```python
from build123d import *

# Parameters (mm, degrees)
F0_W      = 565.15
F0_H      = 1066.8
F1_DEPTH  = 19.05
F3_DEPTH  = 742.95
F5_W      = 304.8
F5_H      = 38.1
F6_DEPTH  = 88.9
F7_W      = 38.1
F7_H      = 806.45
F8_DEPTH  = 88.9
F9_W      = 346.075
F9_H      = 38.1
F10_DEPTH = 88.9
F12_W     = 304.8
F12_H     = 38.1
F13_DEPTH = 88.9
F14_W     = 177.8
F14_H     = 965.2
F15_DEPTH = 38.1


with BuildPart() as f1:
    # F0 (on Top) → F1 (new body)
    with BuildSketch(Plane.XY):
        with Locations((282.575, 533.4)):
            Rectangle(F0_W, F0_H)
    extrude(amount=F1_DEPTH)

    # F2 (on face) → F3 (join)
    with BuildSketch(Plane(origin=(0, 0, 0), x_dir=(1, 0, 0), z_dir=(0, 0, -1))):
        Polygon((130.175, -1016), (130.175, -976.3125), (130.175, -936.625), (50.8, -936.625), (50.8, -1016), align=None)
        Polygon((514.35, -1016), (514.35, -936.625), (434.975, -936.625), (434.975, -976.3125), (434.975, -1016), align=None)
        Polygon((434.975, -50.8), (434.975, -71.4375), (434.975, -109.5375), (434.975, -130.175), (514.35, -130.175), (514.35, -50.8), align=None)
        Polygon((130.175, -71.4375), (130.175, -50.8), (50.8, -50.8), (50.8, -130.175), (130.175, -130.175), (130.175, -109.5375), align=None)
    extrude(amount=F3_DEPTH)

    # F5 (on face) → F6 (join)
    with BuildSketch(Plane(origin=(0, 0, 0), x_dir=(1, 0, 0), z_dir=(0, 0, -1))):
        with Locations((282.575, -90.4875)):
            Rectangle(F5_W, F5_H)
        with Locations((282.575, -976.3125)):
            Rectangle(F5_W, F5_H)
    extrude(amount=F6_DEPTH)

    # F7 (on face) → F8 (join)
    with BuildSketch(Plane(origin=(0, 0, 0), x_dir=(1, 0, 0), z_dir=(0, 0, -1))):
        with Locations((474.6625, -533.4)):
            Rectangle(F7_W, F7_H)
        with Locations((90.4875, -533.4)):
            Rectangle(F7_W, F7_H)
    extrude(amount=F8_DEPTH)

    # F9 (on face) → F10 (join)
    with BuildSketch(Plane(origin=(0, 0, 0), x_dir=(1, 0, 0), z_dir=(0, 0, -1))):
        with Locations((282.575, -533.4)):
            Rectangle(F9_W, F9_H)
    extrude(amount=F10_DEPTH)

    # F12 (on offset) → F13 (join)
    with BuildSketch(Plane(origin=(0, 0, -590.55), x_dir=(1, 0, 0), z_dir=(0, 0, -1))):
        with Locations((282.575, -90.4875)):
            Rectangle(F12_W, F12_H)
        with Locations((282.575, -976.3125)):
            Rectangle(F12_W, F12_H)
    extrude(amount=F13_DEPTH)

    # F14 (on offset) → F15 (join)
    with BuildSketch(Plane(origin=(0, 0, -590.55), x_dir=(1, 0, 0), z_dir=(0, 0, -1))):
        with Locations((219.075, -533.4)):
            Rectangle(F14_W, F14_H)
    extrude(amount=-F15_DEPTH)


solid = f1.part
```
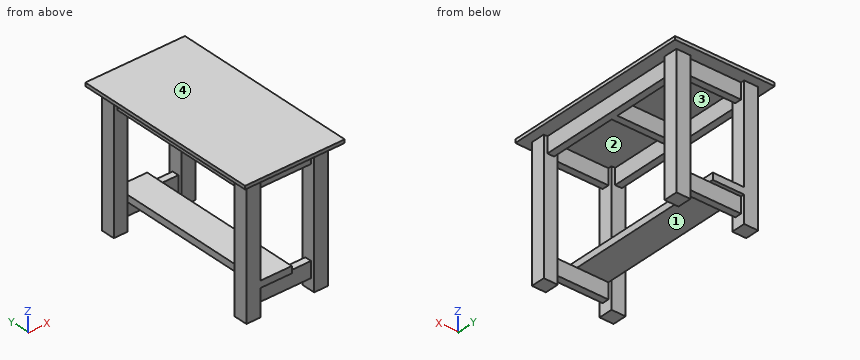
Verification items for the finished model (mm, model axes). Face numbers are marked on the shaded views. Round coordinates to 2 decimals unless told otherwise and drop trailing zeros. Write each loop counter-clockwise with the first axis right and the second up, starting at its lowest first coordinate (ties: lowest second). Pieces come first, ordered by that corner, then holes.
1. Section check B-B on z = -569. Enter the section's corners in (x, y) (3 decimals), plus the area to 3 significant figures.
2. Section check D-D on z = -291. Enter the section's corners in (x, y) (3 decimals).
3. Draft check along Z on the marked faces 1, 2, 3 and 4. Enter one of: +Z half, -Z half, draft (parallel to the pull), parting line (faces both ways), or undercut.
4. Section check A-A on x = 260.5. Enter the section's corners in (y, z).
5. Gauge pin test, flat ends, axial feed: P1, Ø10.5, axis at x = 233.5, y = 56, coming from the -Z side; P2, Ø6, axis at x = 86, z = -306, coming from the -Y side; P3, Ø24, axis at y = 89, z = -375.5, coming from the -X side. Record the tip position at first contact, or that the pin passes through.
6. Scan lines: L1, parallel to X at y = 496.5, z = -80.5; L2, parallel to Y at x = 51, z = -273 (3 decimals); L3, parallel to Z at x = 275, y = 668. Record each from-to range of solid material in increasing order.
Answer:
1. outline: (50.8, 50.8) - (307.975, 50.8) - (307.975, 1016) - (50.8, 1016) - (50.8, 936.625) - (130.175, 936.625) - (130.175, 130.175) - (50.8, 130.175) - close; (434.975, 50.8) - (514.35, 50.8) - (514.35, 130.175) - (434.975, 130.175) - close; (434.975, 936.625) - (514.35, 936.625) - (514.35, 1016) - (434.975, 1016) - close
1. area: 197,000 mm2
2. outline: (50.8, 50.8) - (130.175, 50.8) - (130.175, 130.175) - (50.8, 130.175) - close; (50.8, 936.625) - (130.175, 936.625) - (130.175, 1016) - (50.8, 1016) - close; (434.975, 50.8) - (514.35, 50.8) - (514.35, 130.175) - (434.975, 130.175) - close; (434.975, 936.625) - (514.35, 936.625) - (514.35, 1016) - (434.975, 1016) - close
3. face 1: -Z half
3. face 2: undercut
3. face 3: undercut
3. face 4: +Z half
4. outline: (0, 0) - (71.44, 0) - (71.44, -88.9) - (109.54, -88.9) - (109.54, 0) - (514.35, 0) - (514.35, -88.9) - (552.45, -88.9) - (552.45, 0) - (957.26, 0) - (957.26, -88.9) - (995.36, -88.9) - (995.36, 0) - (1066.8, 0) - (1066.8, 19.05) - (0, 19.05) - close; (50.8, -590.55) - (71.44, -590.55) - (71.44, -679.45) - (109.54, -679.45) - (109.54, -590.55) - (957.26, -590.55) - (957.26, -679.45) - (995.36, -679.45) - (995.36, -590.55) - (1016, -590.55) - (1016, -552.45) - (50.8, -552.45) - close
5. P1: stops at z = -590.55
5. P2: stops at y = 50.8
5. P3: stops at x = 50.8
6. L1: x = 71.44 to 109.54, 455.61 to 493.71
6. L2: y = 50.8 to 130.175, 936.625 to 1016
6. L3: z = -590.55 to -552.45, 0 to 19.05
